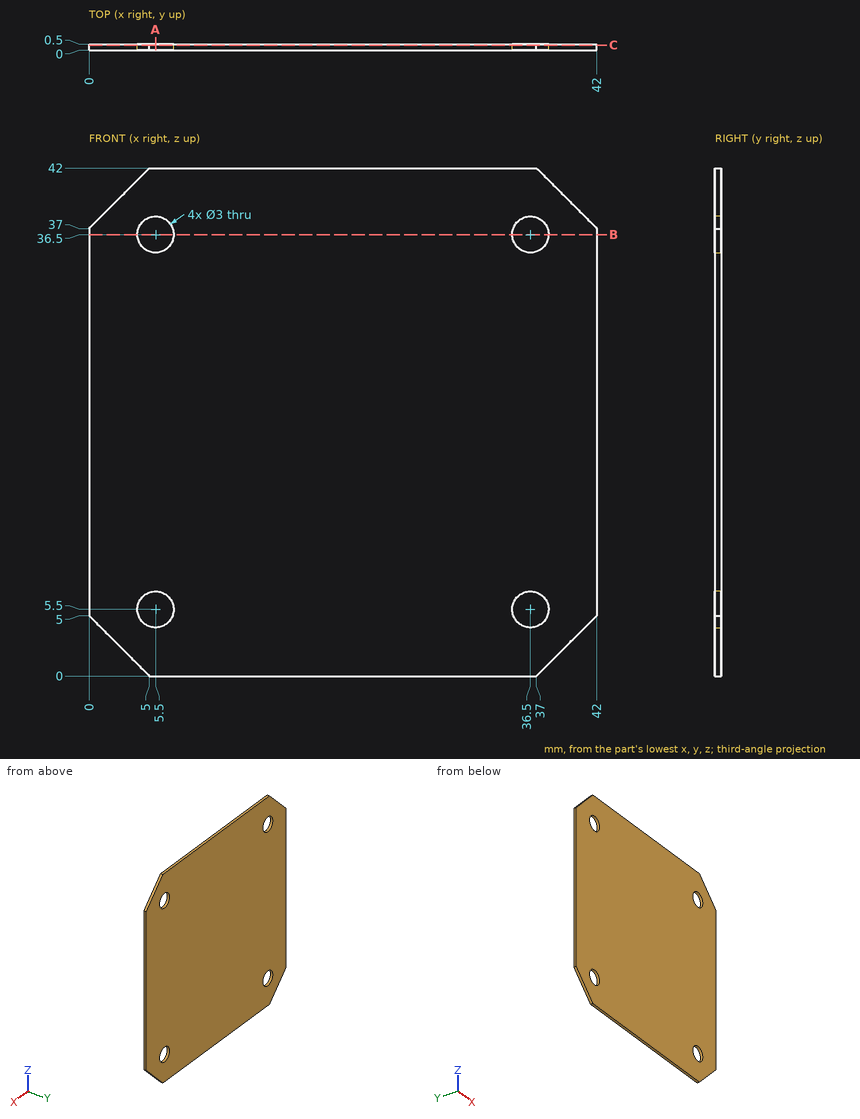
Design review of the part shown in the three views and the two pictorial views. Dimensions are in mm from the part's minimum x, y and z. Round coordinates to 2 decimals unless told otherwise and drop trailing zeros. Write each loop counter-clockwise with the first axis right and the second up, starting at its lowest first coordinate (ties: lowest second). Pieces come first, ordered by that corner, then holes. Notation, with made-up numbers: (68, 45) - (81, 45) arc R19 cw to (81, 58) - close; hole circle Ø3 at (-38, 3.25). An arc over 180 degrees is marked (long way). Return JSON: item names as keys, results as strings. Group by question number.
Item 1: We need section A-A on x = 5.5. Write out the cut boundary in (y, z).
Item 2: We need section C-C on y = 0.4. Write out the cut boundary in (x, z), and give its area (3 significant figures).
Item 3: For probe 1 along X at (y, z) = (0.3, 5.5); probe 2 along X at (y, z) = (0.3, 6); probe 3 along Z at (x, y) = (4.5, 0.1), list the stretches that pass through material, from the lowest coordinate up. Write a range as [from, to].
Item 4: Insertion check: P1, Ø2.5, axis at x = 36.5, z = 36.5, coming from the +Y side. The pin has a flat end and moves straight along its axis. Give the tip position at first contact, or say it passes through.
Item 5: We need section B-B on z = 36.5. Write out the cut boundary in (x, y).
Model answer:
{
 "1": {"outline": "(0, 0) - (0.5, 0) - (0.5, 4) - (0, 4) - close; (0, 7) - (0.5, 7) - (0.5, 35) - (0, 35) - close; (0, 38) - (0.5, 38) - (0.5, 42) - (0, 42) - close"},
 "2": {"outline": "(0, 5) - (5, 0) - (37, 0) - (42, 5) - (42, 37) - (37, 42) - (5, 42) - (0, 37) - close; hole circle Ø3 at (5.5, 5.5); hole circle Ø3 at (5.5, 36.5); hole circle Ø3 at (36.5, 5.5); hole circle Ø3 at (36.5, 36.5)", "area": "1,690 mm²"},
 "3": {"probe 1": "x = [0, 4], [7, 35], [38, 42]", "probe 2": "x = [0, 4.09], [6.91, 35.09], [37.91, 42]", "probe 3": "z = [0.5, 4.38], [6.62, 35.38], [37.62, 41.5]"},
 "4": {"P1": "passes through"},
 "5": {"outline": "(0, 0) - (4, 0) - (4, 0.5) - (0, 0.5) - close; (7, 0) - (35, 0) - (35, 0.5) - (7, 0.5) - close; (38, 0) - (42, 0) - (42, 0.5) - (38, 0.5) - close"}
}
